Input: part model. Units: mm. Frame: model coordinates. Face numbers are marked on the shaded views. A direction names the side the tool comes from. Round coordinates to 2 decimals unless told otherwise and drop trailing zeros. Order: outer loops, then holes, each group sorted by start corner. A loop starts at its lowest first (then second) coordinate and runs counter-clockwise, first axis right, second up. Notation, with made-up numbers: (-11.5, 1.25) -> (6.5, 1.25) arc R7 ccw to (6.5, 12.25) -> close; hole circle Ø3 at (84.25, 44.25). An arc over 180 degrees is marked (long way). Use a Markdown table: item, result.
from build123d import *

# Parameters (mm, degrees)
F0_R        = 25.25
F0_R_2      = 1.75
F0_R_3      = 13.5
F1_DEPTH    = 4
F0_R_4      = 34.5
F1_FACE_R   = 25.25
F1_FACE_R_2 = 1.75
F1_FACE_R_3 = 13.5
F2_DEPTH    = 2
F3_DEPTH    = 7


with BuildPart() as f1:
    # F0 (on Top) → F1 (new body)
    with BuildSketch(Plane.XY):
        Circle(F0_R)
        with Locations((-18.839942, -10.86825)):
            Circle(F0_R_2, mode=Mode.SUBTRACT)
        with Locations((18.839942, -10.86825)):
            Circle(F0_R_2, mode=Mode.SUBTRACT)
        Circle(F0_R_3, mode=Mode.SUBTRACT)
        with Locations((0, 21.749995)):
            Circle(F0_R_2, mode=Mode.SUBTRACT)
    extrude(amount=-F1_DEPTH)

    # F0 (on Top) + F1_face (on face) → F2 (join)
    with BuildSketch(Plane.XY):
        Circle(F0_R_4)
        Circle(F0_R, mode=Mode.SUBTRACT)
    with BuildSketch(Plane(origin=(0, -9.3e-05, 0), x_dir=(1, 0, 0), z_dir=(0, 0, 1))):
        with Locations((0, 9.3e-05)):
            Circle(F1_FACE_R)
        with Locations((-18.839942, -10.868157)):
            Circle(F1_FACE_R_2, mode=Mode.SUBTRACT)
        with Locations((18.839942, -10.868157)):
            Circle(F1_FACE_R_2, mode=Mode.SUBTRACT)
        with Locations((0, 9.3e-05)):
            Circle(F1_FACE_R_3, mode=Mode.SUBTRACT)
        with Locations((0, 21.750087)):
            Circle(F1_FACE_R_2, mode=Mode.SUBTRACT)
    extrude(amount=F2_DEPTH)

    # F0 (on Top) → F3 (join)
    with BuildSketch(Plane.XY):
        Circle(F0_R_4)
        Circle(F0_R, mode=Mode.SUBTRACT)
    extrude(amount=F3_DEPTH)


solid = f1.part
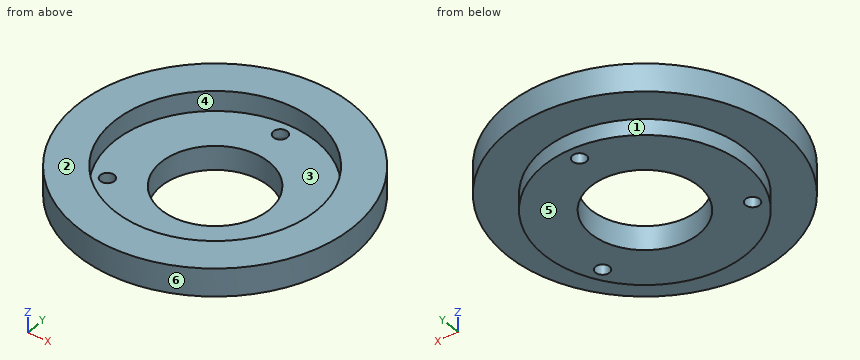
1) Cut plane C-C on x = -23.5. Return loops of the section in (y, z).
Answer key:
| item | result |
|---|---|
| outline | (-25.26, 0) -> (-9.24, 0) -> (-9.24, -4) -> (9.24, -4) -> (9.24, 0) -> (25.26, 0) -> (25.26, 7) -> (9.24, 7) -> (9.24, 2) -> (-9.24, 2) -> (-9.24, 7) -> (-25.26, 7) -> close |
2) Contact query for flat-ended pins moving along their axis: P1, Ø2, axis at y = 13.5, z = -1.5, coming from the +X side; P2, Ø3, axis at y = -19, z = 0, coming from the +X side; P3, Ø4, axis at x = -23.5, z = 3.5, coming from the -Y side. Output: stop coordinate, or through.
Answer key:
| item | result |
|---|---|
| P1 | stops at x = 21.94 |
| P2 | stops at x = 29.73 |
| P3 | stops at y = -26.98 |
3) Cut plane B-B on z = -2. Return loops of the section in (x, y), and give its area (3 significant figures).
Answer key:
| item | result |
|---|---|
| outline | circle Ø50.5 at (0, 0); hole circle Ø3.5 at (-18.84, -10.87); hole circle Ø27 at (0, 0); hole circle Ø3.5 at (0, 21.75); hole circle Ø3.5 at (18.84, -10.87) |
| area | 1,400 mm^2 |
4) Set-up query: the marked faces 1 and 2. Return all of +Z, -Z, +X, -X, +Y, -Y with unobstructed straight access to the full face (end or side cutting, diameter ignored); none if empty.
Answer key:
| item | result |
|---|---|
| face 1 | -Z |
| face 2 | +Z, +X, -X, +Y, -Y |
5) Ray query, probe 1 along Y at (x, z) = (0, -3); probe 2 along Z at (x, y) = (9, 19.5); probe 3 along Z at (x, y) = (22.5, -12.5). Return the intervals inside material, ascending.
Answer key:
| item | result |
|---|---|
| probe 1 | y = -25.25 to -13.5, 13.5 to 20, 23.5 to 25.25 |
| probe 2 | z = -4 to 2 |
| probe 3 | z = 0 to 7 |
6) Cut plane D-D on y = 27.5. Return loops of the section in (x, z), and give its area (3 significant figures).
Answer key:
| item | result |
|---|---|
| outline | (-20.83, 0) -> (20.83, 0) -> (20.83, 7) -> (-20.83, 7) -> close |
| area | 292 mm^2 |
7) Cut plane A-A on y = 0. Return loops of the section in (x, z).
Answer key:
| item | result |
|---|---|
| outline | (-34.5, 0) -> (-25.25, 0) -> (-25.25, -4) -> (-13.5, -4) -> (-13.5, 2) -> (-25.25, 2) -> (-25.25, 7) -> (-34.5, 7) -> close; (13.5, -4) -> (25.25, -4) -> (25.25, 0) -> (34.5, 0) -> (34.5, 7) -> (25.25, 7) -> (25.25, 2) -> (13.5, 2) -> close |
8) Draft query along X for the marked faces 3, 4, 5 and 6. Return one class per face: released by +X, released by -X, zero draft, split by the parting line, or undercut.
Answer key:
| item | result |
|---|---|
| face 3 | undercut |
| face 4 | undercut |
| face 5 | zero draft |
| face 6 | split by the parting line |
